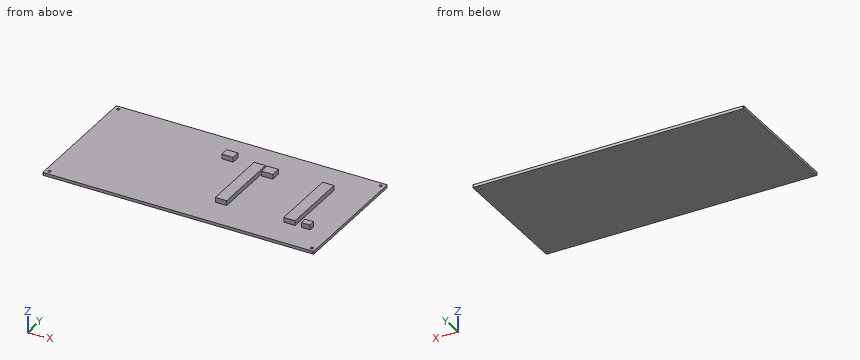
from build123d import *

# Parameters (mm, degrees)
F0_W      = 190
F0_H      = 90.933
F1_DEPTH  = 2
F2_R      = 1
F3_DEPTH  = 2.001
F6_R      = 0.5
F7_W      = 8
F7_H      = 48
F7_H_2    = 7
F8_DEPTH  = 3.4
F9_W      = 8
F9_H      = 6
F10_DEPTH = 3.4


# Not quite as in the source:
# - a feature names something its author has since deleted; it is built from what else it names


with BuildPart() as f1:
    # F0 (on Top) → F1 (new body)
    with BuildSketch(Plane.XY):
        with Locations((95, 45.4665)):
            Rectangle(F0_W, F0_H)
    extrude(amount=F1_DEPTH)

    # F2 (on face) → F3 (cut, through all)
    with BuildSketch(Plane.XY.offset(2)):
        with Locations((3, 87.933)):
            Circle(F2_R)
        with Locations((3, 3)):
            Circle(F2_R)
    f3 = extrude(amount=-F3_DEPTH, mode=Mode.SUBTRACT)

    # F5: F3 across plane
    add(f3.mirror(Plane(origin=(95, 45.4665, 1), x_dir=(0, -1, 0), z_dir=(-1, 0, 0))), mode=Mode.SUBTRACT)

    # F6
    f6_edges = [f1.edges().sort_by_distance(p)[0] for p in [
        (190, 0, 1),
        (190, 90.933, 1),
        (0, 90.933, 1),
        (0, 0, 1),
    ]]
    fillet(f6_edges, radius=F6_R)

    # F7 (on face) → F8 (join)
    with BuildSketch(Plane.XY.offset(2)):
        with Locations((113, 45.233)):
            Rectangle(F7_W, F7_H)
        with Locations((161, 45.233)):
            Rectangle(F7_W, F7_H)
        with Locations((122, 65.733)):
            Rectangle(F7_W, F7_H_2)
        Polygon((169.4320317507, 25.7526094498), (169.4320317507, 21.2526094498), (175.4320317507, 21.2526094498), (175.4320317507, 25.6957146213), align=None)
    extrude(amount=F8_DEPTH)

    # F9 (on face) → F10 (join)
    with BuildSketch(Plane.XY.offset(2)):
        with Locations((91, 70.933)):
            Rectangle(F9_W, F9_H)
    extrude(amount=F10_DEPTH)


solid = f1.part
CAD build for the part. Positions are in the model's coordinates, mm. Coordinates: 2 decimals unless noted, no trailing zeros. Order: outer loops, then holes, each group sorted by start corner. A loop starts at its lowest first (then second) coordinate and runs counter-clockwise, first axis right, second up. Notation, with made-up numbers: (78.5, -9) -> (104.5, -9) arc R22 ccw to (104.5, 30) -> close; hole circle Ø4 at (1.25, 34). An arc over 180 degrees is marked (long way). Answer in a Markdown table with one row per item.
1) Drill centre lines: line 1 (Y direction, x = 3, z = 1.05); line 2 (X direction, y = 69, z = 4.65); line 3 (X direction, y = 33.5, z = 2.5). Where is each one in solid material? Low to high.
Check values:
| item | result |
|---|---|
| line 1 | 0 to 2, 4 to 86.93, 88.93 to 90.93 |
| line 2 | 87 to 95, 109 to 117, 118 to 126, 157 to 165 |
| line 3 | 109 to 117, 157 to 165 |
2) Band-saw the part on A-A (x = 122.5). List the corners of the cut face in (y, z), and give its area (3 significant figures).
Check values:
| item | result |
|---|---|
| outline | (0, 0) -> (90.93, 0) -> (90.93, 2) -> (69.23, 2) -> (69.23, 5.4) -> (62.23, 5.4) -> (62.23, 2) -> (0, 2) -> close |
| area | 206 mm2 |
3) Flat gauge pins, fed straight in: P1, Ø1.7, axis at x = 112, z = 3.5, coming from the +Y side; P2, Ø1.7, axis at x = 114.5, z = 4.5, coming from the -Y side; P3, Ø1.7, axis at y = 50, z = 3, coming from the +X side. Where does each tip first touch, or does it go through?
Check values:
| item | result |
|---|---|
| P1 | y = 69.23 |
| P2 | y = 21.23 |
| P3 | x = 165 |
4) Band-saw the part on C-C (y = 77). List the corners of the cut face in (x, z), and give its area (3 significant figures).
Check values:
| item | result |
|---|---|
| outline | (0, 0) -> (190, 0) -> (190, 2) -> (0, 2) -> close |
| area | 380 mm2 |
5) Band-saw the part on D-D (x = 42.5). List the corners of the cut face in (y, z), and give its area (3 significant figures).
Check values:
| item | result |
|---|---|
| outline | (0, 0) -> (90.93, 0) -> (90.93, 2) -> (0, 2) -> close |
| area | 182 mm2 |
6) Band-saw the part on B-B (y = 33). List the corners of the cut face in (x, z), and give its area (3 significant figures).
Check values:
| item | result |
|---|---|
| outline | (0, 0) -> (190, 0) -> (190, 2) -> (165, 2) -> (165, 5.4) -> (157, 5.4) -> (157, 2) -> (117, 2) -> (117, 5.4) -> (109, 5.4) -> (109, 2) -> (0, 2) -> close |
| area | 434 mm2 |
